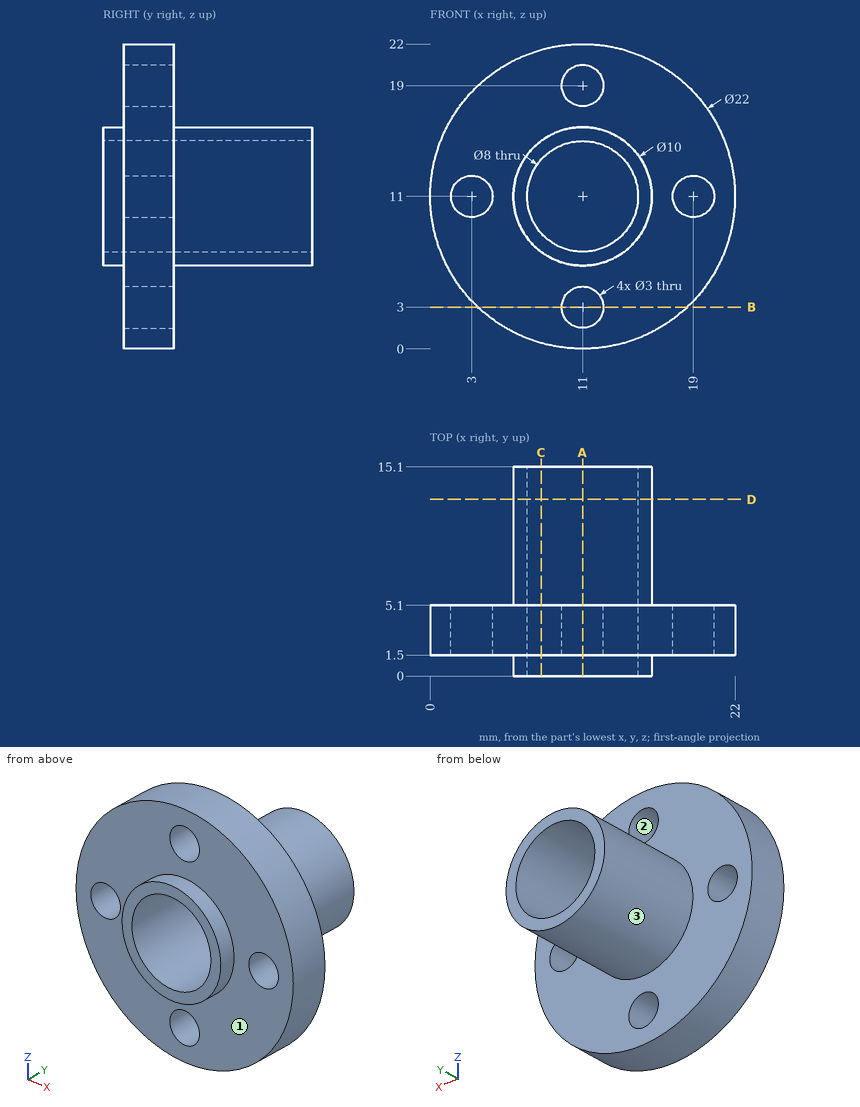
Drawing for the job (mm, zero at the part's lowest x, y, z). A direction names the side the tool comes from. Round coordinates to 2 decimals unless told otherwise and drop trailing zeros. Loops run counter-clockwise (first coordinate to the right, second up) from the corner with the lowest first, then second, coordinate; pieces in that order, holes last. Notation, with made-up numbers: (31.5, 72.25) -> (36.5, 72.25) arc R35 cw to (36.5, 106.25) -> close; hole circle Ø4 at (89, -24). An arc over 180 degrees is marked (long way). Use one line per item in the form item = value. Start each with the question number.
Item 1: Band-saw the part on A-A (x = 11). List the corners of the cut face in (y, z).
Item 2: Drop flat-ended pins along their axis: pin 1 Ø10 at (x, z) = (18.5, 19.5) entering from +Y; pin 2 Ø9 at (x, z) = (11, 11) entering from -Y; pin 3 Ø4 at (x, y) = (5.5, 8) entering from -Z; pin 4 Ø5 at (x, z) = (18, 6) entering from -Y. Give the stop position or say it passes through.
Item 3: Band-saw the part on D-D (y = 12.75). List the corners of the cut face in (x, z), plus the area to 3 significant figures.
Item 4: Tool access for the marked faces 1, 2 and 3: list every direction of +Z, -Z, +X, -X, +Y, -Y with a clear straight run to the whole face (end or side of a thin tool).
Item 5: Band-saw the part on B-B (z = 3). List the corners of the cut face in (x, y).
Item 6: Drill centre lines: line 1 along X through (y, z) = (12.25, 11); line 2 along Y through (x, z) = (15.25, 19.25); line 3 along X through (y, z) = (4.5, 3). Where is each one in solid material? Low to high.
Item 7: Band-saw the part on C-C (x = 8). List the corners of the cut face in (y, z), plus the area to 3 significant figures.
Data:
q1.outline = (0, 6) -> (1.5, 6) -> (1.5, 4.5) -> (5.1, 4.5) -> (5.1, 6) -> (15.1, 6) -> (15.1, 7) -> (0, 7) -> close; (0, 15) -> (15.1, 15) -> (15.1, 16) -> (5.1, 16) -> (5.1, 17.5) -> (1.5, 17.5) -> (1.5, 16) -> (0, 16) -> close; (1.5, 0) -> (5.1, 0) -> (5.1, 1.5) -> (1.5, 1.5) -> close; (1.5, 20.5) -> (5.1, 20.5) -> (5.1, 22) -> (1.5, 22) -> close
q2.pin_1 = 5.1
q2.pin_2 = 0
q2.pin_3 = 7.43
q2.pin_4 = 1.5
q3.outline = circle Ø10 at (11, 11); hole circle Ø8 at (11, 11)
q3.area = 28.3 mm^2
q4.face_1 = -Y
q4.face_2 = +Y, -Y
q4.face_3 = +Y
q5.outline = (3.45, 1.5) -> (9.5, 1.5) -> (9.5, 5.1) -> (3.45, 5.1) -> close; (12.5, 1.5) -> (18.55, 1.5) -> (18.55, 5.1) -> (12.5, 5.1) -> close
q6.line_1 = 6 to 7, 15 to 16
q6.line_2 = 1.5 to 5.1
q6.line_3 = 3.45 to 9.5, 12.5 to 18.55
q7.outline = (0, 7) -> (1.5, 7) -> (1.5, 0.42) -> (5.1, 0.42) -> (5.1, 7) -> (15.1, 7) -> (15.1, 8.35) -> (0, 8.35) -> close; (0, 13.65) -> (15.1, 13.65) -> (15.1, 15) -> (5.1, 15) -> (5.1, 21.58) -> (1.5, 21.58) -> (1.5, 15) -> (0, 15) -> close
q7.area = 88.3 mm^2
